Source: CAD feature listing. Evaluate the final solid. Frame: model axes, mm. Face numbers are marked on the shaded views. A direction names the side the tool comes from. Coordinates: 2 decimals unless noted, no trailing zeros. Loops run counter-clockwise (first coordinate to the right, second up) from the corner with the lowest first, then second, coordinate; pieces in that order, holes last.
Item 1: Section query C-C, the plane y = -4.5. Return the cut outline in (x, z).
Item 2: Line query: probe 1 along Z at (x, y) = (0, -0.6) (3 decimals); probe 2 along Y at (x, z) = (-1.75, 1); probe 3 along Z at (x, y) = (-1.5, -0.75). Output: solid intervals per line, ascending.
Item 3: Section query B-B, the plane x = 0. Return the cut outline in (y, z) (3 decimals).
Item 4: Section query D-D, the plane y = 0.75. Return the cut outline in (x, z).
Item 5: Pull-direction query (X, two-part tool) for the marked faces 3 and 4; classes: +X half, -X half, draft (parallel to the pull), parting line (faces both ways), or undercut.
Item 6: Reachability of the marked faces 1 and 2 from +Z, -Z, +X, -X, +Y, -Y: full face, straight path, thin tool, end or side. Return the list, or none.
Item 7: Section query A-A, the plane z = 0. Return the cut outline in (x, y) (3 decimals).
Item 8: Pin query (flat end, axial travel): pin 1 Ø5 at (x, z) = (-0.5, 1) entering from +Y; pin 2 Ø3 at (x, y) = (4.5, 0) entering from -Z; pin 3 Ø2 at (y, z) = (-0.5, -5) entering from +X. Return the tip coordinate at first contact, or that it passes through.
Autodesk Inventor part; units mm, degrees
ref_plane "YZ Plane" through (0, 0, 0) normal (1, 0, 0) x (0, 1, 0)
ref_plane "XZ Plane" through (0, 0, 0) normal (0, 1, 0) x (-1, 0, 0)
ref_plane "XY Plane" through (0, 0, 0) normal (0, 0, 1) x (1, 0, 0)
sketch "Boceto1" plane through (0, 0, 0) normal (0, 1, 0) x (-1, 0, 0)
  circle A0 centre (0, 0) radius 7
  dimension "d0" = 14
extrude "Extrusión1" add sketch "Boceto1" along normal blind 2
sketch "Boceto2" plane through (0, 0, 0) normal (0, -1, 0) x (1, 0, 0)
  circle A0 centre (0, 0) radius 5.625
  circle A1 centre (0, 0) radius 7
  dimension "d3" = 11.25
  dimension "d4" = 14
extrude "Extrusión2" add sketch "Boceto2" along normal blind 2.5
sketch "Boceto3" plane through (0, 0, 0) normal (0, -1, 0) x (1, 0, 0)
  line L0 (0, 0) -> (2.8, 0)
  line L1 (2.8, 0) -> (2.8, -1.4)
  line L2 (2.8, -1.4) -> (1.4, -1.4)
  line L3 (1.4, -1.4) -> (1.4, -2.8)
  line L4 (1.4, -2.8) -> (-1.4, -2.8)
  line L5 (-1.4, -2.8) -> (-1.4, -1.4)
  line L6 (-1.4, -1.4) -> (-2.8, -1.4)
  line L7 (-2.8, -1.4) -> (-2.8, 1.4)
  line L8 (-2.8, 1.4) -> (-1.4, 1.4)
  line L9 (-1.4, 1.4) -> (-1.4, 2.8)
  line L10 (-1.4, 2.8) -> (1.4, 2.8)
  line L11 (1.4, 2.8) -> (1.4, 1.4)
  line L12 (1.4, 1.4) -> (2.8, 1.4)
  line L13 (2.8, 1.4) -> (2.8, 0)
  line L14 (-1.4, 1.4) -> (1.4, 1.4)
  line L15 (1.4, 1.4) -> (1.4, -1.4)
  line L16 (1.4, -1.4) -> (-1.4, -1.4)
  line L17 (-1.4, -1.4) -> (-1.4, 1.4)
  line L18 (-1.4, 1.4) -> (1.4, 1.4)
  line L19 (1.4, 1.4) -> (1.4, -1.4)
  line L20 (1.4, -1.4) -> (-1.4, -1.4)
  line L21 (-1.4, -1.4) -> (-1.4, 1.4)
  dimension "d7" = 2.8
  dimension "d8" = 1.4
  dimension "d9" = 1.4
  dimension "d10" = 1.4
  dimension "d11" = 2.8
  dimension "d12" = 1.4
  dimension "d13" = 1.4
  dimension "d14" = 2.8
  dimension "d15" = 1.4
  dimension "d16" = 1.4
  dimension "d17" = 2.8
  dimension "d18" = 1.4
  dimension "d19" = 1.4
extrude "Extrusión3" add sketch "Boceto3" along normal blind 5 contours L15 L16 L17 L14
sketch "Boceto8" plane through (0, 2, 0) normal (0, 1, 0) x (1, 0, 0)
  circle A0 centre (0, 0) radius 6
  dimension "d55" = 12
extrude "Extrusión6" cut sketch "Boceto8" against normal blind 1
fillet "Empalme2" radius 1 3 edges at (-6, 1, 0) (-6, 2, 0) (7, 2, 0)
fillet "Empalme5" radius 1 4 edges at (1.4, -2.5, 1.4) (-1.4, -2.5, 1.4) (1.4, -2.5, -1.4) (-1.4, -2.5, -1.4)
properties part number "Boton Tapa"
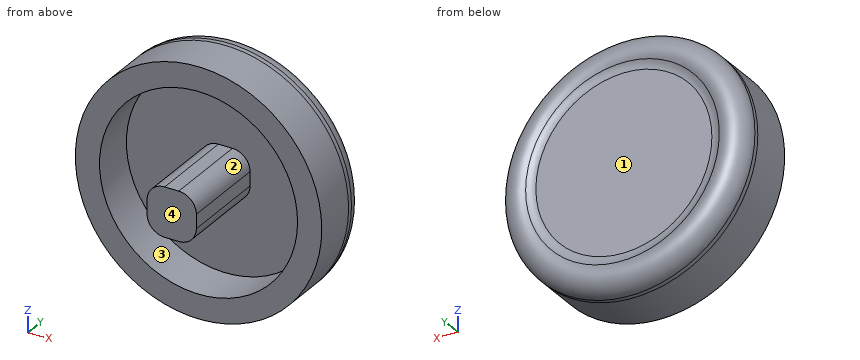
Verdict:
1. outline: (-1.4, -0.4) arc R1 ccw to (-0.4, -1.4) - (0.4, -1.4) arc R1 ccw to (1.4, -0.4) - (1.4, 0.4) arc R1 ccw to (0.4, 1.4) - (-0.4, 1.4) arc R1 ccw to (-1.4, 0.4) - close
2. probe 1: z = -7 to -5.625, -1.4 to 1.4, 5.625 to 7
2. probe 2: y = 0 to 1
2. probe 3: z = -6.84 to -5.42, 5.42 to 6.84
3. outline: (-5, -1.4) - (0, -1.4) - (0, -5.625) - (-2.5, -5.625) - (-2.5, -7) - (0.268, -7) arc R1 ccw to (1.134, -5.5) arc R1 cw to (1, -5) - (1, 5) arc R1 cw to (1.134, 5.5) arc R1 ccw to (0.268, 7) - (-2.5, 7) - (-2.5, 5.625) - (0, 5.625) - (0, 1.4) - (-5, 1.4) - close
4. outline: circle Ø13.75 at (0, 0)
5. face 3: undercut
5. face 4: draft
6. face 1: +Y
6. face 2: -Y
7. outline: (-7, -2.5) - (-5.625, -2.5) - (-5.625, 0) - (-1.4, 0) - (-1.4, -5) - (1.4, -5) - (1.4, 0) - (5.625, 0) - (5.625, -2.5) - (7, -2.5) - (7, 0.268) arc R1 ccw to (5.5, 1.134) arc R1 cw to (5, 1) - (-5, 1) arc R1 cw to (-5.5, 1.134) arc R1 ccw to (-7, 0.268) - close
8. pin 1: stops at y = 1
8. pin 2: stops at z = -6.32
8. pin 3: stops at x = 5.74
